Part model, mm, in its own coordinate system. Face numbers are marked on the shaded views. A direction names the side the tool comes from. Give positions to 0.01 mm unless a question says otherwise; leave off trailing zeros. Order: outer loops, then holes, each group sorted by start corner. A loop starts at its lowest first (then second) coordinate and runs counter-clockwise, first axis right, second up.
1. Slice it at C-C on x = 14.5. List the corners of the cut face in (y, z), and give its area (3 significant figures).
2. Drop a flat-ended pin along its axis: pin 1 Ø1.5 at (x, z) = (-16, -3.5) entering from -Y. Give the stop position or say it passes through.
3. Which spindle directions (+Z, -Z, +X, -X, +Y, -Y) get a long thin tool onto all of the face, cutting with end or side? Do the marked faces 4, 5 and 6. Say none if no direction does.
4. Mould opens along Y. For the marked faces 1, 2 and 3 say: +Y half, -Y half, draft (parallel to the pull), parting line (faces both ways), or undercut.
5. Slice it at A-A on z = -0.5. List the corners of the cut face in (x, y).
6. Probe line 1 (Z direction, x = 5.5, y = 37.5); line 2 (Y direction, x = -14.5, z = -2.7); line 3 (Y direction, x = -16.5, z = -4.7). List the from-to ranges inside material, lowest first.
7. Slice it at B-B on x = 2.5. List the corners of the cut face in (y, z).
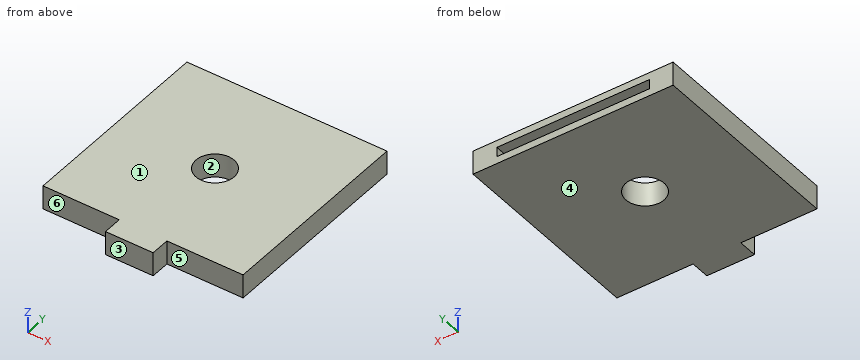
Autodesk Inventor part; units mm, degrees
ref_plane "YZ Plane" through (0, 0, 0) normal (1, 0, 0) x (0, 1, 0)
ref_plane "XZ Plane" through (0, 0, 0) normal (0, 1, 0) x (-1, 0, 0)
ref_plane "XY Plane" through (0, 0, 0) normal (0, 0, 1) x (1, 0, 0)
sketch "Sketch1" plane through (0, 0, 0) normal (0, 0, 1) x (1, 0, 0)
  line L0 (-8.9346, 3.531) -> (-24.9346, 3.531)
  line L1 (-24.9346, 3.531) -> (-24.9346, 45.531)
  line L2 (-24.9346, 45.531) -> (17.0654, 45.531)
  line L3 (17.0654, 45.531) -> (17.0654, 3.531)
  line L4 (17.0654, 3.531) -> (1.0654, 3.531)
  line L5 (-8.9346, -0.469) -> (1.0654, -0.469)
  line L6 (-8.9346, 3.531) -> (-8.9346, -0.469)
  line L7 (1.0654, 3.531) -> (1.0654, -0.469)
  circle A0 centre (-3.9346, 24.531) radius 4
  point P0 (0, 0)
extrude "Extrusion4" add sketch "Sketch1" against normal blind 5
sketch "Sketch3" plane through (-24.9346, 45.531, 0) normal (0, 1, 0) x (1, 0, 0)
  line L0 (0, 0) -> (0, 5)
  line L1 (16, 5) -> (0, 5)
  line L2 (5, 3.5) -> (5, 1.5)
  line L3 (0, 0) -> (16, 0)
  line L4 (5, 3.5) -> (37, 3.5)
  line L5 (5, 1.5) -> (37, 1.5)
  line L6 (37, 3.5) -> (37, 1.5)
  point P0 (24.9346, 0)
extrude "Extrusion6" cut sketch "Sketch3" against normal blind 10
properties part number "suport cu rulment pentru tija" material "Gold"
Data:
1. outline: (3.53, -5) - (45.53, -5) - (45.53, 0) - (3.53, 0) - close
1. area: 210 mm2
2. pin 1: stops at y = 3.53
3. face 4: -Z, +X, -X, +Y, -Y
3. face 5: +Z, -Z, +X, -Y
3. face 6: +Z, -Z, -X, -Y
4. face 1: draft
4. face 2: undercut
4. face 3: -Y half
5. outline: (-24.93, 3.53) - (-8.93, 3.53) - (-8.93, -0.47) - (1.07, -0.47) - (1.07, 3.53) - (17.07, 3.53) - (17.07, 45.53) - (-24.93, 45.53) - close; hole circle Ø8 at (-3.93, 24.53)
6. line 1: z = -5 to -3.5, -1.5 to 0
6. line 2: y = 3.53 to 35.53
6. line 3: y = 3.53 to 45.53
7. outline: (3.53, -5) - (45.53, -5) - (45.53, -3.5) - (35.53, -3.5) - (35.53, -1.5) - (45.53, -1.5) - (45.53, 0) - (3.53, 0) - close
